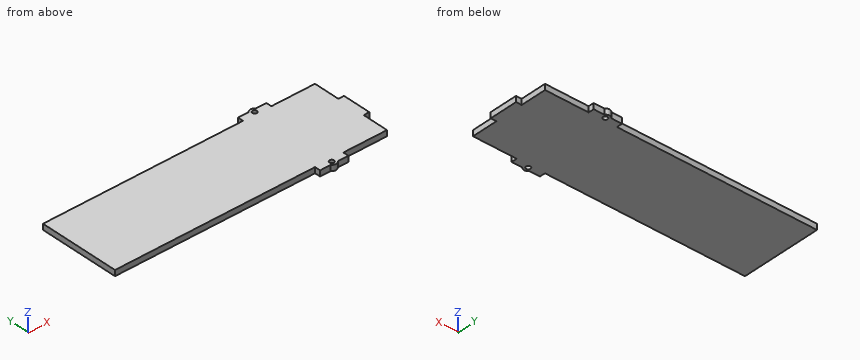
from build123d import *

# Parameters (mm, degrees)
SKETCH1_W           = 102
SKETCH1_H           = 71
BOSS_EXTRUDE1_DEPTH = 5
SKETCH3_W           = 25
SKETCH3_H           = 5
SKETCH3_W_2         = 5
SKETCH3_H_2         = 25
BOSS_EXTRUDE2_DEPTH = 5
SKETCH4_R           = 2
CUT_EXTRUDE1_DEPTH  = 5
SKETCH5_R           = 4
SKETCH5_R_2         = 2
BOSS_EXTRUDE3_DEPTH = 5
SKETCH6_W           = 138
SKETCH6_H           = 71
BOSS_EXTRUDE4_DEPTH = 5


with BuildPart() as part:
    # Sketch1 → Boss-Extrude1 (new body)
    with BuildSketch(Plane.XY):
        Rectangle(SKETCH1_W, SKETCH1_H)
    extrude(amount=BOSS_EXTRUDE1_DEPTH)

    # Sketch3 → Boss-Extrude2 (add)
    with BuildSketch(Plane.XY.offset(5)):
        with Locations((0, 38)):
            Rectangle(SKETCH3_W, SKETCH3_H)
        with Locations((53.5, 0)):
            Rectangle(SKETCH3_W_2, SKETCH3_H_2)
        with Locations((0, -38)):
            Rectangle(SKETCH3_W, SKETCH3_H)
    extrude(amount=-BOSS_EXTRUDE2_DEPTH)

    # Sketch4 → Cut-Extrude1 (cut)
    with BuildSketch(Plane.XY.offset(5)):
        with Locations((0, 38)):
            Circle(SKETCH4_R)
        with Locations((0, -38)):
            Circle(SKETCH4_R)
    extrude(amount=-CUT_EXTRUDE1_DEPTH, mode=Mode.SUBTRACT)

    # Sketch5 → Boss-Extrude3 (add)
    # profile 1 of 2: a face of its own
    with BuildSketch(Plane.XY.offset(5)):
        with Locations((0, 38)):
            Circle(SKETCH5_R)
        with Locations((0, 38)):
            Circle(SKETCH5_R_2, mode=Mode.SUBTRACT)
    # profile 2 of 2: a face of its own
    with BuildSketch(Plane.XY.offset(5)):
        with Locations((0, -38)):
            Circle(SKETCH5_R)
        with Locations((0, -38)):
            Circle(SKETCH5_R_2, mode=Mode.SUBTRACT)
    extrude(amount=-BOSS_EXTRUDE3_DEPTH)

    # Sketch6 → Boss-Extrude4 (add)
    with BuildSketch(Plane.XY.offset(5)):
        with Locations((-120, 0)):
            Rectangle(SKETCH6_W, SKETCH6_H)
    extrude(amount=-BOSS_EXTRUDE4_DEPTH)


solid = part.part
Read the model definition and answer for the solid it produces. Units are mm, in the model's axes. Coordinates: 2 decimals unless noted, no trailing zeros. Loops run counter-clockwise (first coordinate to the right, second up) from the corner with the lowest first, then second, coordinate; pieces in that order, holes last.
Q1. Each of these flat-tipped pins is pushed along its axis until it touches: pin 1 Ø2.5 at (x, z) = (6.5, 2.5) entering from +Y; pin 2 Ø1.5 at (y, z) = (38, 2) entering from +X; pin 3 Ø2 at (x, z) = (-64, 2) entering from -Y. Where does it stop, or does it pass through?
Q2. Consider probe 1 along Y at (x, z) = (0, 1.4); probe 2 along X at (y, z) = (-31, 1.3); probe 3 along Y at (x, z) = (-145, 2.2). Determine where each line is inside the solid, lowest interval first.
Q3. The part is cut by section B-B on x = -19. Write down the section's boundary in (y, z).
Q4. The part is cut by section A-A on z = 3.6. Write down the section's boundary in (x, y), and give its area (3 significant figures).
Results below:
1. pin 1: stops at y = 40.5
1. pin 2: stops at x = 12.5
1. pin 3: stops at y = -35.5
2. probe 1: y = -42 to -40, -36 to 36, 40 to 42
2. probe 2: x = -189 to 51
2. probe 3: y = -35.5 to 35.5
3. outline: (-35.5, 0) - (35.5, 0) - (35.5, 5) - (-35.5, 5) - close
4. outline: (-189, -35.5) - (-12.5, -35.5) - (-12.5, -40.5) - (-3.12, -40.5) arc R4 ccw to (3.12, -40.5) - (12.5, -40.5) - (12.5, -35.5) - (51, -35.5) - (51, -12.5) - (56, -12.5) - (56, 12.5) - (51, 12.5) - (51, 35.5) - (12.5, 35.5) - (12.5, 40.5) - (3.12, 40.5) arc R4 ccw to (-3.12, 40.5) - (-12.5, 40.5) - (-12.5, 35.5) - (-189, 35.5) - close; hole circle Ø4 at (0, -38); hole circle Ø4 at (0, 38)
4. area: 17,400 mm2
